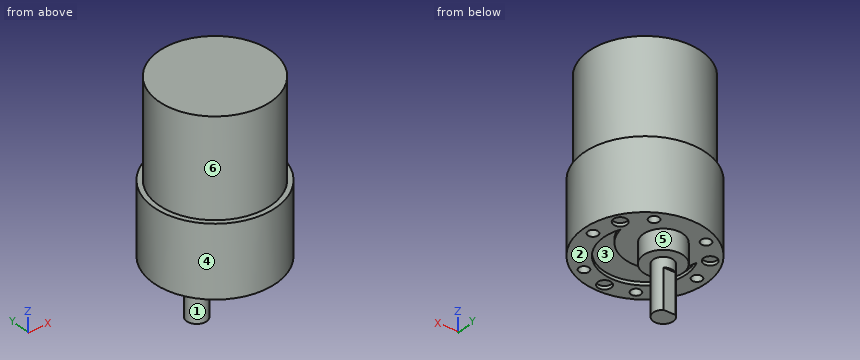
```python
from build123d import *

# Parameters (mm, degrees)
SKETCH_1_R          = 18.5
EXTRUDE_1_DEPTH     = 21.5
SKETCH_2_R          = 17
EXTRUDE_2_DEPTH     = 29.4
CUT_EXTRUDE_1_DEPTH = 1
SKETCH_4_R          = 6
EXTRUDE_3_DEPTH     = 6
SKETCH_5_R          = 3
EXTRUDE_4_DEPTH     = 15
CUT_EXTRUDE_START   = -12
CUT_EXTRUDE_2_DEPTH = 12
SKETCH_7_R          = 1.5
CUT_EXTRUDE_3_DEPTH = 5
SKETCH_8_R          = 2
CUT_EXTRUDE_4_DEPTH = 1


with BuildPart() as part:
    # 草图1 → 凸台-拉伸1 (new body)
    with BuildSketch(Plane.XY):
        Circle(SKETCH_1_R)
    extrude(amount=EXTRUDE_1_DEPTH)

    # 草图2 → 凸台-拉伸2 (add)
    with BuildSketch(Plane.XY.offset(21.5)):
        Circle(SKETCH_2_R)
    extrude(amount=EXTRUDE_2_DEPTH)

    # 草图3 → 切除-拉伸1 (cut)
    with BuildSketch(Plane(origin=(0, 0, 0), x_dir=(-1, 0, 0), z_dir=(0, 0, -1))):
        with BuildLine():
            ThreePointArc((-11.36051163, 5.214285714), (0, -4.5), (11.36051163, 5.214285714))
            ThreePointArc((11.36051163, 5.214285714), (0, -12.5), (-11.36051163, 5.214285714))
        make_face()
    extrude(amount=-CUT_EXTRUDE_1_DEPTH, mode=Mode.SUBTRACT)

    # 草图4 → 凸台-拉伸3 (add)
    with BuildSketch(Plane(origin=(0, 0, 0), x_dir=(-1, 0, 0), z_dir=(0, 0, -1))):
        with Locations(Location((0, 7, 0), (0, 0, 180))):
            Circle(SKETCH_4_R)
    extrude(amount=EXTRUDE_3_DEPTH)

    # 草图5 → 凸台-拉伸4 (add)
    with BuildSketch(Plane(origin=(0, 0, -6), x_dir=(-1, 0, 0), z_dir=(0, 0, -1))):
        with Locations((0, 7)):
            Circle(SKETCH_5_R)
    extrude(amount=EXTRUDE_4_DEPTH)

    # 草图6 → 切除-拉伸2 (cut)
    with BuildSketch(Plane(origin=(0, 0, -21), x_dir=(-1, 0, 0), z_dir=(0, 0, -1)).offset(CUT_EXTRUDE_START)):
        with BuildLine():
            Line((0, 9.4), (1.8, 9.4))
            ThreePointArc((1.8, 9.4), (0, 10), (-1.8, 9.4))
            Line((-1.8, 9.4), (0, 9.4))
        make_face()
    extrude(amount=CUT_EXTRUDE_2_DEPTH, mode=Mode.SUBTRACT)

    # 草图7 → 切除-拉伸3 (cut)
    with BuildSketch(Plane(origin=(0, 0, 0), x_dir=(-1, 0, 0), z_dir=(0, 0, -1))):
        with Locations((15.5, 0)):
            Circle(SKETCH_7_R)
        with Locations(Location((-15.5, 0, 0), (0, 0, 180))):
            Circle(SKETCH_7_R)
        with Locations((-7.75, -13.423393759)):
            Circle(SKETCH_7_R)
        with Locations(Location((7.75, 13.423393759, 0), (0, 0, 180))):
            Circle(SKETCH_7_R)
        with Locations((-7.75, 13.423393759)):
            Circle(SKETCH_7_R)
        with Locations(Location((7.75, -13.423393759, 0), (0, 0, 180))):
            Circle(SKETCH_7_R)
    extrude(amount=-CUT_EXTRUDE_3_DEPTH, mode=Mode.SUBTRACT)

    # 草图8 → 切除-拉伸4 (cut)
    with BuildSketch(Plane(origin=(0, 0, 0), x_dir=(-1, 0, 0), z_dir=(0, 0, -1))):
        with Locations((0, -15.5)):
            Circle(SKETCH_8_R)
        with Locations((-13.423393759, 7.75)):
            Circle(SKETCH_8_R)
        with Locations((13.423393759, 7.75)):
            Circle(SKETCH_8_R)
    extrude(amount=-CUT_EXTRUDE_4_DEPTH, mode=Mode.SUBTRACT)


solid = part.part
```
Design review of the part built by this model. Coordinates are the model's own, in mm. Face numbers are marked on the shaded views. A direction names the side the tool comes from. Give positions to 0.01 mm unless a question says otherwise; leave off trailing zeros. Order: outer loops, then holes, each group sorted by start corner. A loop starts at its lowest first (then second) coordinate and runs counter-clockwise, first axis right, second up. Notation, with made-up numbers: (42, 5) - (65, 5) arc R23 ccw to (65, 18) - close; hole circle Ø7 at (9, 62.5). An arc over 180 degrees is marked (long way). Use a Markdown table: item, result. Add a question column.
(1) Add section C-C on z = -2.5. Give the boundary of the cut face in (x, y).
(2) Add section D-D on x = 7. Give the boundary of the cut face in (y, z), then the cut area to 3 significant figures.
(3) Clearance check with flat-ended pins moving along their axes: P1, Ø3.5, axis at x = -7.5, y = 13.5, coming from the -Z side; P2, Ø12, axis at y = 1, z = 6.5, coming from the +X side; P3, Ø1.5, axis at x = 7.5, y = -14, coming from the -Z side; P4, Ø2, axis at x = 3.5, z = 19, coming from the -Y side. State where each tip first meets the part, or that it passes through.
(4) Add section A-A on x = 0. Give the boundary of the cut face in (y, z).
(5) Machinability: for the marked faces 4, 5 and 6, which of the approach directions +Z, -Z, +X, -X, +Y, -Y give a long, thin tool a straight path to every point of the face, cutting with its end or side? Answer none if there is none.
(6) Wall thickness on probe 1 along Y at (x, z) = (-8.5, 2); probe 2 along Y at (x, z) = (-7.75, 2.45); probe 3 along Z at (x, y) = (-0.5, -5.5): over which ranges is each line inside the solid? List them lowest first. Write a range as [from, to].
(7) Mouldability with a two-part tool opening along Y and no side actions: class the marked faces 1, 2 and 3 as +Y half, -Y half, draft (parallel to the pull), parting line (faces both ways), or undercut.
(8) Add section B-B on y = -3. Give the boundary of the cut face in (x, z).
Report:
| question | item | result |
|---|---|---|
| 1 | outline | circle Ø12 at (0, 7) |
| 2 | outline | (-17.12, 0) - (-14.72, 0) - (-14.72, 5) - (-12.12, 5) - (-12.12, 0) - (-10.36, 0) - (-10.36, 1) - (-2.12, 1) - (-2.12, 0) - (12.12, 0) - (12.12, 5) - (14.72, 5) - (14.72, 0) - (17.12, 0) - (17.12, 21.5) - (15.49, 21.5) - (15.49, 50.9) - (-15.49, 50.9) - (-15.49, 21.5) - (-17.12, 21.5) - close |
| 2 | area | 1,610 mm² |
| 3 | P1 | stops at z = 0 |
| 3 | P2 | stops at x = 18.5 |
| 3 | P3 | stops at z = 5 |
| 3 | P4 | stops at y = -18.33 |
| 4 | outline | (-18.5, 0) - (-17.5, 0) - (-17.5, 1) - (-13.5, 1) - (-13.5, 0) - (-12.5, 0) - (-12.5, 1) - (-4.5, 1) - (-4.5, 0) - (1, 0) - (1, -6) - (4, -6) - (4, -21) - (9.4, -21) - (9.4, -9) - (10, -9) - (10, -6) - (13, -6) - (13, 0) - (18.5, 0) - (18.5, 21.5) - (17, 21.5) - (17, 50.9) - (-17, 50.9) - (-17, 21.5) - (-18.5, 21.5) - close |
| 5 | face 4 | +Z, -Z |
| 5 | face 5 | -Z |
| 5 | face 6 | +Z |
| 6 | probe 1 | y = [-16.43, -14.72], [-12.12, 12.12], [14.72, 16.43] |
| 6 | probe 2 | y = [-16.8, -14.92], [-11.92, 11.92], [14.92, 16.8] |
| 6 | probe 3 | z = [1, 50.9] |
| 7 | face 1 | parting line |
| 7 | face 2 | draft |
| 7 | face 3 | undercut |
| 8 | outline | (-18.26, 0) - (-12.13, 0) - (-12.13, 1) - (-5.68, 1) - (-5.68, 0) - (5.68, 0) - (5.68, 1) - (12.13, 1) - (12.13, 0) - (18.26, 0) - (18.26, 21.5) - (16.73, 21.5) - (16.73, 50.9) - (-16.73, 50.9) - (-16.73, 21.5) - (-18.26, 21.5) - close |
